```python
from build123d import *

# Parameters (mm, degrees)
SKETCH1_W                    = 96.0628
SKETCH1_H                    = 90.3478
PCB_DEPTH                    = 1.6256
SKETCH5_R                    = 1.5875
PCB_HOLES_DEPTH              = 66.957101229
PCI_104_CONNECTOR_DEPTH      = 9.2964
PCI_104_CONNECTOR_DEPTH_BACK = 12.6238
SKETCH2_W                    = 7.9756
SKETCH2_H                    = 60.2234
SKETCH6_W                    = 65.278
SKETCH6_H                    = 7.366
SKETCH6_W_2                  = 46.9138
SKETCH6_H_2                  = 9.398
PCB_EDGE_CONNS_DEPTH         = 5.461
HEAT_SINK_DEPTH              = 14.5288
SKETCH8_W                    = 12.578663299
SKETCH8_H                    = 5.969
SKETCH8_W_2                  = 12.468978526
CUT_EXTRUDE1_DEPTH           = 5.6388
SKETCH9_W                    = 24.13
SKETCH9_H                    = 8.89
CUT_EXTRUDE2_DEPTH           = 14.5288
SKETCH10_W                   = 15.661416919
SKETCH10_H                   = 4.637831463
SKETCH10_W_2                 = 10.456810418
SKETCH10_H_2                 = 2.475294653
SKETCH10_W_3                 = 2.739234778
SKETCH10_H_3                 = 53.34
BOSS_EXTRUDE1_DEPTH          = 5.08
SKETCH11_R                   = 0.504502566
BOSS_EXTRUDE2_DEPTH          = 1.27
LPATTERN1_COUNT              = 6
LPATTERN1_PITCH              = 2.54
LPATTERN1_COUNT_DIR2         = 2
LPATTERN1_PITCH_DIR2         = 2.54
SKETCH12_R                   = 0.464941127
BOSS_EXTRUDE3_DEPTH          = 1.27
LPATTERN2_COUNT              = 4
LPATTERN2_PITCH              = 2.54
SKETCH13_R                   = 0.853348332
BOSS_EXTRUDE4_DEPTH          = 1.27
LPATTERN3_COUNT              = 21
LPATTERN3_PITCH              = 2.54


with BuildPart() as part:
    # Sketch1 → PCB (new body)
    with BuildSketch(Plane.XY):
        Rectangle(SKETCH1_W, SKETCH1_H)
    extrude(amount=PCB_DEPTH)

    # Sketch5 → PCB_Holes (cut, through all)
    with BuildSketch(Plane.XY.offset(1.6256)):
        with Locations((-42.7736, 36.83)):
            Circle(SKETCH5_R)
        with Locations((42.9514, 40.005)):
            Circle(SKETCH5_R)
        with Locations((42.9514, -40.005)):
            Circle(SKETCH5_R)
        with Locations((-42.7736, -36.83)):
            Circle(SKETCH5_R)
    extrude(amount=-PCB_HOLES_DEPTH, mode=Mode.SUBTRACT)

    # Sketch2 → PCI-104_Connector (add, two sides: drawn at the far end of the back side and taken through both)
    with BuildSketch(Plane.XY.offset(1.6256).offset(-PCI_104_CONNECTOR_DEPTH_BACK)):
        with Locations((-39.6494, 0.4064)):
            Rectangle(SKETCH2_W, SKETCH2_H)
    extrude(amount=PCI_104_CONNECTOR_DEPTH + PCI_104_CONNECTOR_DEPTH_BACK)

    # Sketch6 → PCB_Edge_Conns (add)
    with BuildSketch(Plane.XY.offset(1.6256)):
        with Locations((-6.9342, -46.0629)):
            Rectangle(SKETCH6_W, SKETCH6_H)
        with Locations((-15.9385, 45.0469)):
            Rectangle(SKETCH6_W_2, SKETCH6_H_2)
    extrude(amount=PCB_EDGE_CONNS_DEPTH)

    # Sketch7 → Heat Sink (add)
    with BuildSketch(Plane.XY.offset(1.6256)):
        Polygon((32.7914, 37.6555), (-32.929016802, 37.6555), (-32.929016802, 39.8145), (-45.507680101, 39.8145), (-45.507680101, 33.8455), (-35.347680101, 33.8455), (-35.347680101, -33.8455), (-45.681124108, -33.8455), (-45.681124108, -39.8145), (32.7914, -39.8145), align=None)
    extrude(amount=HEAT_SINK_DEPTH)

    # Sketch8 → Cut-Extrude1 (cut)
    with BuildSketch(Plane.XY.offset(16.1544)):
        with Locations((-39.218348452, 36.83)):
            Rectangle(SKETCH8_W, SKETCH8_H)
        with Locations((-39.446634845, -36.83)):
            Rectangle(SKETCH8_W_2, SKETCH8_H)
    extrude(amount=-CUT_EXTRUDE1_DEPTH, mode=Mode.SUBTRACT)

    # Sketch9 → Cut-Extrude2 (cut)
    with BuildSketch(Plane.XY.offset(16.1544)):
        with Locations((6.130519899, 33.2105)):
            Rectangle(SKETCH9_W, SKETCH9_H)
    extrude(amount=-CUT_EXTRUDE2_DEPTH, mode=Mode.SUBTRACT)

    # Sketch10 → Boss-Extrude1 (add)
    with BuildSketch(Plane.XY.offset(1.6256)):
        with Locations((6.040104986, 31.44690823)):
            Rectangle(SKETCH10_W, SKETCH10_H)
        with Locations((32.684734403, -43.337331173)):
            Rectangle(SKETCH10_W_2, SKETCH10_H_2)
        with Locations((44.95848031, -9.569270887)):
            Rectangle(SKETCH10_W_3, SKETCH10_H_3)
    extrude(amount=BOSS_EXTRUDE1_DEPTH)

    # Sketch11 → Boss-Extrude2 (add)
    with BuildSketch(Plane.XY.offset(6.7056)):
        with Locations((12.839671728, 30.359366813)):
            Circle(SKETCH11_R)
    boss_extrude2 = extrude(amount=BOSS_EXTRUDE2_DEPTH)

    # LPattern1: Boss-Extrude2 6 × 2
    with Locations(*[(-i * LPATTERN1_PITCH, j * LPATTERN1_PITCH_DIR2, 0) for i in range(LPATTERN1_COUNT) for j in range(LPATTERN1_COUNT_DIR2) if (i, j) != (0, 0)]):
        add(boss_extrude2)

    # Sketch12 → Boss-Extrude3 (add)
    with BuildSketch(Plane.XY.offset(6.7056)):
        with Locations(Location((36.988776709, -43.465687533, 0), (0, 0, 180))):
            Circle(SKETCH12_R)
    boss_extrude3 = extrude(amount=BOSS_EXTRUDE3_DEPTH)

    # LPattern2: Boss-Extrude3 ×4
    with Locations(*[(-i * LPATTERN2_PITCH, 0, 0) for i in range(1, LPATTERN2_COUNT)]):
        add(boss_extrude3)

    # Sketch13 → Boss-Extrude4 (add)
    with BuildSketch(Plane.XY.offset(6.7056)):
        with Locations(Location((44.932694638, -34.705275196, 0), (0, 0, 180))):
            Circle(SKETCH13_R)
    boss_extrude4 = extrude(amount=BOSS_EXTRUDE4_DEPTH)

    # LPattern3: Boss-Extrude4 ×21
    with Locations(*[(0, i * LPATTERN3_PITCH, 0) for i in range(1, LPATTERN3_COUNT)]):
        add(boss_extrude4)


solid = part.part
```
Model file for the job. Use its own axes, mm. A direction names the side the tool comes from. Coordinates: 2 decimals unless noted, no trailing zeros. Write each loop counter-clockwise with the first axis right and the second up, starting at its lowest first coordinate (ties: lowest second). Pieces come first, ordered by that corner, then holes. Notation, with made-up numbers: (-25.5, 29.25) - (-20.5, 29.25) arc R29 ccw to (-20.5, 56.25) - close; hole circle Ø5 at (50.25, 83). An arc over 180 degrees is marked (long way). Use a Markdown table: item, result. Add a question column.
Item 1: Two-plate mould, pull along X, no slides. Class faces 4 (the face through (46.328, -10, 4)), 5 (the face through (-41.26, -36.35, 0.82)), 6 (the face through (-16, 40.348, 4)): pulls with the +X half, pulls with the -X half, needs draft (parallel to the pull), parting line crosses it, or undercut.
Item 2: Band-saw the part on C-C, the plane z = -5.25. Write the cut outline in (x, y).
Item 3: Band-saw the part on A-A, the plane x = 19.5. Write the cut outline in (y, z).
Item 4: 3-axis set-ups, long thin cutter, end or side, ignore diameter. For faces 1 (the face through (-45.681, -37, 6)), 2 (the face through (-40, -33.846, 6)), 3 (the face through (25.705, -46, 4)): which of +Z, -Z, +X, -X, +Y, -Y reach the whole face in a straight line?
Item 5: Band-saw the part on B-B, the plane y = 21.5. Write the cut outline in (x, z), and give its area (3 significant figures).
Item 6: Band-saw the part on D-D, the plane x = -28.5. Write the cut outline in (y, z).
Item 7: Drill centre lines: line 1 along Y through (x, z) = (-38, 9); line 2 along X through (y, z) = (-4.5, 1.75); line 3 along X through (y, z) = (29.5, 10). Where is each one in solid material? Low to high.
Item 8: Drop flat-ended pins along their axis: pin 1 (1.9 mm diameter, centred on x = 45, y = -7, fed in from +Z); pin 2 (10 mm diameter, centred on x = 26.5, z = 5.5, fed in from +Y); pin 3 (6.5 mm diameter, centred on y = 37.5, z = 7, fed in from -X). Give the stop position or say it passes through.
A:
| question | item | result |
|---|---|---|
| 1 | face 4 | pulls with the +X half |
| 1 | face 5 | undercut |
| 1 | face 6 | needs draft |
| 2 | outline | (-43.64, -29.71) - (-35.66, -29.71) - (-35.66, 30.52) - (-43.64, 30.52) - close |
| 3 | outline | (-49.75, 1.63) - (-45.17, 1.63) - (-45.17, 0) - (45.17, 0) - (45.17, 1.63) - (37.66, 1.63) - (37.66, 16.15) - (-39.81, 16.15) - (-39.81, 1.63) - (-42.38, 1.63) - (-42.38, 7.09) - (-49.75, 7.09) - close |
| 4 | face 1 | +Z, -X, +Y, -Y |
| 4 | face 2 | +Z, -X |
| 4 | face 3 | +Z, -Y |
| 5 | outline | (-48.03, 0) - (-43.64, 0) - (-43.64, -11) - (-35.66, -11) - (-35.66, 0) - (48.03, 0) - (48.03, 1.63) - (32.79, 1.63) - (32.79, 16.15) - (-35.35, 16.15) - (-35.35, 1.63) - (-35.66, 1.63) - (-35.66, 10.92) - (-43.64, 10.92) - (-43.64, 1.63) - (-48.03, 1.63) - close |
| 5 | area | 1,310 mm² |
| 6 | outline | (-49.75, 1.63) - (-45.17, 1.63) - (-45.17, 0) - (45.17, 0) - (45.17, 1.63) - (49.75, 1.63) - (49.75, 7.09) - (40.35, 7.09) - (40.35, 1.63) - (37.66, 1.63) - (37.66, 16.15) - (-39.81, 16.15) - (-39.81, 1.63) - (-42.38, 1.63) - (-42.38, 7.09) - (-49.75, 7.09) - close |
| 7 | line 1 | y = -39.81 to -33.85, -29.71 to 30.52, 33.85 to 39.81 |
| 7 | line 2 | x = -43.64 to -35.66, -35.35 to 32.79, 43.59 to 46.33 |
| 7 | line 3 | x = -43.64 to -35.66, -35.35 to -5.93, 18.2 to 32.79 |
| 8 | pin 1 | stops at z = 7.98 |
| 8 | pin 2 | stops at y = 45.17 |
| 8 | pin 3 | stops at x = -45.51 |
